Build history of the part. All positions in model axes, mm. A direction names the side the tool comes from. Coordinates: 2 decimals unless noted, no trailing zeros. Loops run counter-clockwise (first coordinate to the right, second up) from the corner with the lowest first, then second, coordinate; pieces in that order, holes last. Notation, with made-up numbers: M 43,-5 L 95,-5 A12 cw 95,12 Z; hole C 46.25,14.5 d9. An arc over 180 degrees is marked long. Write each question's results on one line, items separated by ' | '. Start each with the question number.
from build123d import *

# Parameters (mm, degrees)
SKETCH1_R        = 2.5
SHAFT_BODY_DEPTH = 36
D_CUT_DEPTH      = 15
FILLET_2_R       = 0.25


with BuildPart() as part:
    # Sketch1 → Shaft Body (new body, symmetric)
    with BuildSketch(Plane.XY):
        Circle(SKETCH1_R)
    extrude(amount=SHAFT_BODY_DEPTH, both=True)

    # Sketch2 → D Cut (cut)
    with BuildSketch(Plane.XY.offset(36)):
        with BuildLine():
            Line((-1.5, 2), (1.5, 2))
            ThreePointArc((1.5, 2), (0, 2.5), (-1.5, 2))
        make_face()
    extrude(amount=-D_CUT_DEPTH, mode=Mode.SUBTRACT)

    # Fillet 2
    fillet_2_edges = [part.edges().sort_by_distance(p)[0] for p in [
        (-1.118033989, -2.236067977, 36),
        (0, 2, 36),
    ]]
    fillet(fillet_2_edges, radius=FILLET_2_R)


solid = part.part
1. Band-saw the part on B-B, the plane z = -28. List the corners of the cut face in (x, y), plus the area to 3 significant figures.
2. Wall check: line 1 along X through (y, z) = (-0.25, -10.5); line 2 along Y through (x, z) = (1.45, -24). Give the ranges that are in metal, low to high.
3. Band-saw the part on A-A, the plane x = 0. List the corners of the cut face in (y, z).
4. Pin check, flat tip, straight feed: pin 1 (1.5 mm diameter, centred on x = -0.5, z = 28.5, fed in from +Y). Stop position of the tip, or through.
5. Which spindle directions (+Z, -Z, +X, -X, +Y, -Y) get a long thin tool onto all of the face, cutting with end or side? Do faces 1 (the flat face through (0, 0, 36)), 2 (the flat face through (0, 2, 28)). Say none if no direction does.
6. Band-saw the part on C-C, the plane z = 27. List the corners of the cut face in (x, y).
Checked values:
1) outline: C 0,0 d5 | area: 19.6 mm²
2) line 1: -2.49 to 2.49 | line 2: -2.04 to 2.04
3) outline: M -2.5,-36 L 2.5,-36 L 2.5,21 L 2,21 L 2,35.75 A0.25 ccw 1.75,36 L -2.25,36 A0.25 ccw -2.5,35.75 Z
4) pin 1: y = 2
5) face 1: +Z, +X, -X, +Y, -Y | face 2: +Z, +X, -X, +Y
6) outline: M -1.5,2 A2.5 ccw long 1.5,2 Z
